```python
from build123d import *

# Parameters (mm, degrees)
SKETCH1_R           = 3.3782
BOSS_EXTRUDE1_DEPTH = 5.588
FILLET1_R           = 50.8
SKETCH2_R           = 3.3782
CUT_EXTRUDE1_DEPTH  = 1260.942692133
FILLET2_R           = 3.175
CUT_EXTRUDE2_DEPTH  = 1255.509228579


with BuildPart() as part:
    # Sketch1 (on Top Plane) → Boss-Extrude1 (new body)
    with BuildSketch(Plane(origin=(0, 0, 0), x_dir=(1, 0, 0), z_dir=(0, 1, 0))):
        Polygon((0, 0), (0, 469.9), (439.7375, 469.9), (439.7375, 773.938), (994.205378114, 773.938), (885.3805, 697.738), (885.3805, 495.45319999), (177.8, 0), align=None)
        with Locations(Location((24.6253, 21.463, 0), (0, 0, 270))):
            Circle(SKETCH1_R, mode=Mode.SUBTRACT)
        with Locations(Location((69.0753, 323.85, 0), (0, 0, 270))):
            Circle(SKETCH1_R, mode=Mode.SUBTRACT)
        with Locations(Location((495.8715, 438.15, 0), (0, 0, 270))):
            Circle(SKETCH1_R, mode=Mode.SUBTRACT)
        with Locations(Location((495.8715, 640.588, 0), (0, 0, 270))):
            Circle(SKETCH1_R, mode=Mode.SUBTRACT)
        with Locations(Location((829.2465, 640.588, 0), (0, 0, 270))):
            Circle(SKETCH1_R, mode=Mode.SUBTRACT)
    extrude(amount=BOSS_EXTRUDE1_DEPTH)

    # Fillet1
    fillet1_edges = [part.edges().sort_by_distance(p)[0] for p in [
        (439.7375, 2.794, -469.9),
    ]]
    fillet(fillet1_edges, radius=FILLET1_R)

    # Sketch2 → Cut-Extrude1 (cut, through all)
    with BuildSketch(Plane(origin=(0, 5.588, 0), x_dir=(1, 0, 0), z_dir=(0, 1, 0))):
        with Locations(Location((31.75, 454.025, 0), (0, 0, 270))):
            Circle(SKETCH2_R)
        with Locations(Location((471.4875, 758.063, 0), (0, 0, 270))):
            Circle(SKETCH2_R)
    extrude(amount=-CUT_EXTRUDE1_DEPTH, mode=Mode.SUBTRACT)

    # Fillet2
    fillet2_edges = [part.edges().sort_by_distance(p)[0] for p in [
        (0, 2.794, 0),
        (0, 2.794, -469.9),
        (439.7375, 2.794, -773.938),
        (994.205378114, 2.794, -773.938),
        (885.3805, 2.794, -697.738),
        (885.3805, 2.794, -495.45319999),
        (177.8, 2.794, 0),
    ]]
    fillet(fillet2_edges, radius=FILLET2_R)

    # Sketch3 → Cut-Extrude2 (cut, through all)
    with BuildSketch(Plane(origin=(0, 5.588, 0), x_dir=(1, 0, 0), z_dir=(0, 1, 0))):
        with BuildLine():
            Line((3.175, 0), (176.798926345, 0))
            ThreePointArc((176.798926345, 0), (177.753667259, 0.146948681), (178.620031531, 0.574192259))
            Line((178.620031531, 0.574192259), (197.577542747, 13.848384519))
            ThreePointArc((197.577542747, 13.848384519), (195.844814203, 12.993897363), (193.935332376, 12.7))
            Line((193.935332376, 12.7), (3.175, 12.7))
            ThreePointArc((3.175, 12.7), (0.92993597, 13.62993597), (0, 15.875))
            Line((0, 15.875), (0, 3.175))
            ThreePointArc((0, 3.175), (0.92993597, 0.92993597), (3.175, 0))
        make_face()
    extrude(amount=-CUT_EXTRUDE2_DEPTH, mode=Mode.SUBTRACT)


solid = part.part
```
The model under review builds one solid part; all positions refer to its coordinate system, in mm. Round coordinates to 2 decimals unless told otherwise and drop trailing zeros. Order: outer loops, then holes, each group sorted by start corner. A loop starts at its lowest first (then second) coordinate and runs counter-clockwise, first axis right, second up.
Item 1: For pin 1 (3 mm diameter, centred on y = 3.5, z = -623, fed in from +X); pin 2 (3 mm diameter, centred on y = 2.5, z = -702, fed in from -X); pin 3 (3 mm diameter, centred on x = 271, z = -335, fed in from -Y); pin 4 (1.7 mm diameter, centred on x = 121, y = 3, fed in from -Z), all flat-tipped, find the tip position at first contact; note any pin that passes through.
Working result:
pin 1: stops at x = 885.38
pin 2: stops at x = 439.74
pin 3: stops at y = 0
pin 4: stops at z = -469.9
Item 2: Add section B-B, the plane x = 167. State the section outline as (y, z) points, and give its area (3 significant figures).
Working result:
outline: (0, -469.9) - (5.59, -469.9) - (5.59, -12.7) - (0, -12.7) - close
area: 2,550 mm2
Item 3: To check wall thickness, follow probe 1 along Z at (x, y) = (48.5, 0.65); probe 2 along X at (y, z) = (3.05, -574); probe 3 along Z at (x, y) = (72, 0.8). State the ranges of each line that lie inside material, in increasing order.
Working result:
probe 1: z = -469.9 to -12.7
probe 2: x = 439.74 to 885.38
probe 3: z = -469.9 to -325.54, -322.16 to -12.7
Item 4: Add section A-A, the plane y = 4.7. Count the separate pieces of the cut face and the enclosed holes in it, and give its area (3 significant figures).
Working result:
separate pieces: 1
enclosed holes: 7
area: 378,000 mm2
Item 5: Add section C-C, the plane z = -122.5. State the section outline as (x, y) points, and give its area (3 significant figures).
Working result:
outline: (0, 0) - (352.75, 0) - (352.75, 5.59) - (0, 5.59) - close
area: 1,970 mm2
